```python
from build123d import *

# Parameters (mm, degrees)
SKETCH1_R           = 2.6375
BOSS_EXTRUDE1_DEPTH = 4


with BuildPart() as part:
    # Sketch1 → Boss-Extrude1 (new body)
    with BuildSketch(Plane(origin=(0, 4, 0), x_dir=(1, 0, 0), z_dir=(0, 1, 0))):
        with BuildLine():
            Line((85.735483712, 77.323980784), (87.547228424, 77.6361992))
            ThreePointArc((87.547228424, 77.6361992), (88.638512401, 78.055387782), (89.486725608, 78.859846695))
            Line((89.486725608, 78.859846695), (90.859907816, 80.800603382))
            ThreePointArc((90.859907816, 80.800603382), (91.392372444, 82.866543385), (90.417013283, 84.763989347))
            ThreePointArc((90.417013283, 84.763989347), (89.660091993, 85.325292733), (88.8112973, 85.73460789))
            ThreePointArc((88.8112973, 85.73460789), (88.035402119, 86.161615284), (87.417993221, 86.796560083))
            ThreePointArc((87.417993221, 86.796560083), (66.977031359, 89.139944323), (66.603972706, 68.568478678))
            ThreePointArc((66.603972706, 68.568478678), (67.327519051, 67.51101449), (67.543844855, 66.248100016))
            ThreePointArc((67.543844855, 66.248100016), (71.92413831, 61.058265048), (77.438126505, 65.022769043))
            ThreePointArc((77.438126505, 65.022769043), (77.298986696, 66.69694337), (76.281652818, 68.033824571))
            Line((76.281652818, 68.033824571), (72.915652336, 70.521815026))
            ThreePointArc((72.915652336, 70.521815026), (72.158360379, 70.866374525), (71.326393596, 70.872979652))
            ThreePointArc((71.326393596, 70.872979652), (69.787994238, 70.962547772), (68.497017033, 71.804018441))
            ThreePointArc((68.497017033, 71.804018441), (68.277664092, 85.314017723), (81.632240885, 87.369127207))
            ThreePointArc((81.632240885, 87.369127207), (82.929152896, 85.595651679), (82.669646853, 83.413942984))
            ThreePointArc((82.669646853, 83.413942984), (82.079827473, 81.296958117), (82.454695982, 79.131551589))
            ThreePointArc((82.454695982, 79.131551589), (83.778317702, 77.652816556), (85.735483712, 77.323980784))
        make_face()
        with Locations((72.538655529, 66.020358214)):
            Circle(SKETCH1_R, mode=Mode.SUBTRACT)
        with Locations((87.073540725, 81.04630307)):
            Circle(SKETCH1_R, mode=Mode.SUBTRACT)
    extrude(amount=-BOSS_EXTRUDE1_DEPTH)


solid = part.part
```
Read the model definition and answer for the solid it produces. Units are mm, in the model's axes. A direction names the side the tool comes from. Coordinates: 2 decimals unless noted, no trailing zeros. Loops run counter-clockwise (first coordinate to the right, second up) from the corner with the lowest first, then second, coordinate; pieces in that order, holes last.
(1) The part is cut by section D-D (z = -82). Determine the outline of the cut face in (x, y), and give its area (3 significant figures).
Solution:
outline: (62.64, 0) - (66.4, 0) - (66.4, 4) - (62.64, 4) - close; (82.17, 0) - (84.61, 0) - (84.61, 4) - (82.17, 4) - close; (89.53, 0) - (91.36, 0) - (91.36, 4) - (89.53, 4) - close
area: 32.2 mm2
(2) The part is cut by section B-B (y = 2.55). Determine the outline of the cut face in (x, z) (1 decimal), and give its area (3 significant figures).
Solution:
outline: (66.6, -68.6) arc R13.9 ccw (long way) to (87.4, -86.8) arc R3 cw to (88.8, -85.7) arc R5 ccw to (90.4, -84.8) arc R3 ccw to (90.9, -80.8) - (89.5, -78.9) arc R3 ccw to (87.5, -77.6) - (85.7, -77.3) arc R3 ccw to (82.5, -79.1) arc R5 ccw to (82.7, -83.4) arc R3 cw to (81.6, -87.4) arc R10.3 cw to (68.5, -71.8) arc R3 cw to (71.3, -70.9) arc R2 ccw to (72.9, -70.5) - (76.3, -68) arc R3 ccw to (77.4, -65) arc R5 ccw to (67.5, -66.2) arc R3 cw to start; hole circle Ø5.3 at (72.5, -66); hole circle Ø5.3 at (87.1, -81)
area: 245 mm2
(3) Consider line 1 along X through (y, z) = (1.3, -81.5); line 2 along X through (y, z) = (1.4, -82.5); line 3 along Z through (x, y) = (89, 0.9). Determine where each line is inside the solid, lowest interval first.
Solution:
line 1: x = 62.52 to 66.25, 82.09 to 84.48, 89.67 to 91.23
line 2: x = 62.77 to 66.59, 82.29 to 84.87, 89.27 to 91.41
line 3: z = -85.66 to -82.85, -79.24 to -78.32
(4) The mould has two halves that part along X. Classify faces 1 (the face through (71.821, 2.028, -61.072)), 2 (the face through (74.62, 2.03, -69.26)), 3 (the face through (70.59, 2.03, -67.8)), 4 (the face through (69.809, 2.028, -70.956)): released by +X, released by -X, zero draft, split by the parting line, or undercut.
Solution:
face 1: split by the parting line
face 2: released by +X
face 3: undercut
face 4: undercut
(5) The part is cut by section A-A (x = 86.5). Determine the outline of the cut face in (y, z).
Solution:
outline: (0, -87.94) - (4, -87.94) - (4, -83.62) - (0, -83.62) - close; (0, -78.47) - (4, -78.47) - (4, -77.46) - (0, -77.46) - close
(6) A tool of negligible diameter and unlimited length cuts with its end or side. For faces 5 (the face through (82.08, 2.03, -81.33)), 6 (the face through (88.625, 2.028, -78.047)), from which of +Z, -Z, +X, -X, +Y, -Y can it reach the whole face along a straight path? Write none if from no direction.
Solution:
face 5: +Y, -Y
face 6: +Z, +X, +Y, -Y
(7) The part is cut by section C-C (x = 72). Determine the outline of the cut face in (y, z), and give its area (3 significant figures).
Solution:
outline: (0, -91.95) - (4, -91.95) - (4, -88.1) - (0, -88.1) - close; (0, -70.89) - (4, -70.89) - (4, -68.6) - (0, -68.6) - close; (0, -63.44) - (4, -63.44) - (4, -61.05) - (0, -61.05) - close
area: 34.2 mm2
(8) Flat-ended cylindrical pins translate along their axes: pin 1 Ø4 at (x, z) = (79, -89) entering from -Y; pin 2 Ø3 at (x, z) = (87.07, -81.05) entering from -Y; pin 3 Ø1.5 at (x, y) = (71.5, 1.5) entering from -Z; pin 4 Ø1 at (y, z) = (1, -72) entering from -X. Find the tip coordinate at first contact, or state that the pin passes through.
Solution:
pin 1: stops at y = 0
pin 2: passes through
pin 3: stops at z = -92.03
pin 4: stops at x = 63.69
